Work out the finished part from the listing and answer in its coordinate system (mm). Face numbers are marked on the shaded views. A direction names the side the tool comes from. Round coordinates to 2 decimals unless told otherwise and drop trailing zeros. Loops run counter-clockwise (first coordinate to the right, second up) from the corner with the lowest first, then second, coordinate; pieces in that order, holes last. Notation, with made-up numbers: (15.25, -25.5) - (35.25, -25.5) arc R4 ccw to (35.25, -18.5) - close; hole circle Ø2 at (14, 53.25). An arc over 180 degrees is marked (long way). Answer as CSV lines item,"result". Start each with the question number.
Q1. Section D-D on z = -5.08 is taken. Count the separate pieces of the cut face and the enclosed holes in it, then the cut area to 3 significant figures.
Q2. Straight lines are drawn through the part: L1, parallel to Y at x = -4.75, z = -5.08; L2, parallel to Y at x = -4, z = -5.08; L3, parallel to X at y = 70, z = -1.5. For each, find the intervals that lie inside material, in ascending order. Write a range as [from, to].
Q3. Each of these flat-tipped pins is pushed along its axis until it touches: pin 1 Ø7.5 at (y, z) = (10.5, -10) entering from -X; pin 2 Ø6 at (x, z) = (-13, -13.5) entering from -Y; pin 3 Ø6 at (y, z) = (50, -3) entering from -X. Where does it stop, or does it pass through?
Q4. For the marked faces 1, 2 and 3, determine the directions among +Z, -Z, +X, -X, +Y, -Y from which every point of the face is accessible in a straight line to the end or side of a thin tool.
Q5. Section A-A on x = -3 is taken. Write down the section's boundary in (y, z).
Q6. Section C-C on x = -13.25 is taken. Write down the section's boundary in (y, z).
Autodesk Inventor part; units mm, degrees
ref_plane "Work Plane2" through (0, 17.6708, -22.228) normal (0, 0, -1) x (0, 1, 0)
ref_plane "YZ Plane" through (0, 0, 0) normal (1, 0, 0) x (0, 1, 0)
ref_plane "XZ Plane" through (0, 0, 0) normal (0, 1, 0) x (-1, 0, 0)
ref_plane "Work Plane1" through (0, 0, 0) normal (0, 0, 1) x (1, 0, 0)
sketch "Sketch1" plane through (0, 0, 0) normal (0, 0, 1) x (1, 0, 0)
  arc A0 (18.9992, 41.108) -> (0, 60.0877) centre (-0.0008, 41.0877) ccw construction
  arc A1 (0, 22.1284) -> (18.9992, 41.108) centre (-0.0008, 41.1284) ccw construction
  arc A2 (44.3468, 60.0877) -> (25.3476, 41.108) centre (44.3476, 41.0877) ccw construction
  arc A3 (25.3476, 41.108) -> (44.3468, 22.1284) centre (44.3476, 41.1284) ccw construction
  line L0 (10.16, 73.6386) -> (5.7912, 73.6386) construction
  line L1 (0, 77.677) -> (0, 67.7202) construction
  line L2 (5.7912, 73.6386) -> (13.9012, 73.6386) construction
  line L3 (-25.35, 77.677) -> (-25.35, 84.027)
  line L4 (-25.35, -6.35) -> (-25.35, 0)
  line L5 (-25.35, 77.677) -> (-25.35, 0) construction
  arc A4 (-6.0324, 64.4924) -> (-6.0325, 17.7644) centre (-0.0008, 41.1284) ccw
  arc A5 (-6.0324, 64.4924) -> (-6.0325, 17.7644) centre (-0.0008, 41.1284) ccw
  arc A6 (-0.0008, 60.1276) -> (-0.0008, 22.1292) centre (-0.0008, 41.1284) ccw
  line L6 (-6.0324, 64.4924) -> (-6.0324, 73.6386)
  line L7 (-6.0324, 73.6386) -> (-0.0008, 73.6385)
  line L8 (10.16, 8.5775) -> (5.7912, 8.5775) construction
  line L9 (-6.0325, 8.5775) -> (-0.0008, 8.5775)
  line L10 (-6.0325, 8.5775) -> (-6.0325, 17.7644)
  line L11 (-0.0008, 73.6385) -> (-0.0008, 60.1276)
  line L12 (-0.0008, 8.5775) -> (-0.0008, 22.1292)
  point P0 (0, 0)
  dimension "d12" = 18.9992
  dimension "d13" = 24.13
  dimension "d19" = 6.0317
  dimension "d22" = 6.0317
  dimension "d23" = 0
  dimension "d24" = 0
ref_plane "Work Plane2" through (0, 17.6708, -22.228) normal (0, 0, -1) x (0, 1, 0)
extrude "Extrusion1" add sketch "Sketch1" against normal up to surface (22.228 mm away)
sketch "Sketch2" plane through (-6.0324, 64.4924, 0) normal (-1, 0, 0) x (0, 0, 1)
  circle A0 centre (-17.148, 5.715) radius 1.9304
  circle A1 centre (-5.08, 5.715) radius 1.9304
  circle A2 centre (-5.08, -50.0243) radius 1.9304
  circle A3 centre (-17.148, -50.0243) radius 1.9304
  point P0 (0, -64.4924)
extrude "Extrusion2" cut sketch "Sketch2" along normal mid plane 25.4
fillet "Fillet1" radius 3.175 1 edges at (-6.0324, 64.4924, -11.114)
fillet "Fillet2" radius 3.175 1 edges at (-6.0325, 17.7644, -11.114)
equation "\"d19\" = d18"
properties part number "motor mount cap-10"
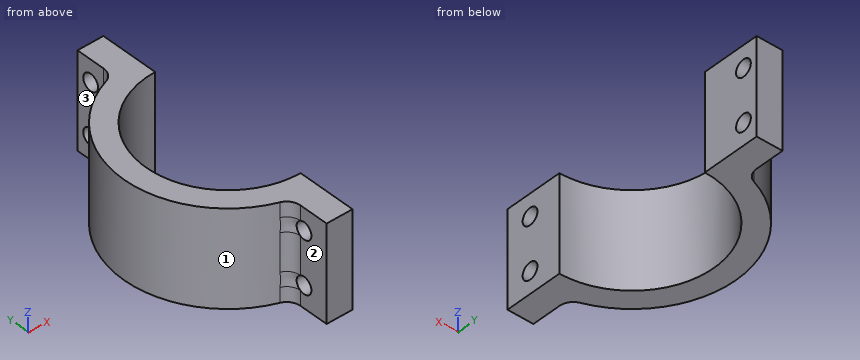
Findings:
1,separate pieces,"3"
1,enclosed holes,"0"
1,area,"407 mm^2"
2,L1,"y = [8.58, 12.54], [16.4, 22.73], [59.52, 68.28], [72.14, 73.64]"
2,L2,"y = [8.58, 12.54], [16.4, 22.55], [59.7, 68.28], [72.14, 73.64]"
2,L3,"x = [-6.03, 0]"
3,pin 1,"stops at x = -6.03"
3,pin 2,"stops at y = 19.17"
3,pin 3,"stops at x = -23.41"
4,face 1,"+Z, -Z, -X"
4,face 2,"+Z, -Z, -X, -Y"
4,face 3,"+Z, -Z, -X, +Y"
5,outline,"(8.58, -22.23) - (22.37, -22.23) - (22.37, 0) - (8.58, 0) - close; (59.89, -22.23) - (73.64, -22.23) - (73.64, 0) - (59.89, 0) - close; hole circle Ø3.86 at (14.47, -17.15); hole circle Ø3.86 at (14.47, -5.08); hole circle Ø3.86 at (70.21, -17.15); hole circle Ø3.86 at (70.21, -5.08)"
6,outline,"(20.96, -22.23) - (27.51, -22.23) - (27.51, 0) - (20.96, 0) - close; (54.75, -22.23) - (61.3, -22.23) - (61.3, 0) - (54.75, 0) - close"
